Geometry: see drawing. Coordinates: mm, zero at the bounding-box minimum. A direction names the side the tool comes from. Give positions to 0.01 mm unless a question says otherwise; leave off trailing zeros. Loops run counter-clockwise (first coordinate to the right, second up) from the corner with the lowest first, then second, coordinate; pieces in that order, holes last. Notation, with made-up numbers: (38.5, 75) -> (78.5, 75) arc R17 cw to (78.5, 108) -> close; hole circle Ø9 at (46.25, 75.5). An arc over 180 degrees is marked (long way). Return JSON: item names as keys, results as strings. Group by question number.
(1) Cut plane C-C on z = 1.2. Return loops of the section in (x, y) (1 decimal), then the cut area to 3 significant figures.
(2) Cut plane D-D on x = 3.5. Return loops of the section in (y, z), then the cut area to 3 significant figures.
(3) Cut plane A-A on y = 21. Return loops of the section in (x, z) (1 decimal).
(4) Cut plane B-B on x = 24. Return loops of the section in (y, z) (1 decimal).
(5) Access query for the marked faces 1, 2, 3 and 4. Directions: +Z, -Z, +X, -X, +Y, -Y. A direction counts if a zero-diameter tool reaches every point of the face in a straight line with its end or side. Return the directions, or none.
(6) Draft query along X for the marked faces 5 and 6. Return one class per face: released by +X, released by -X, zero draft, split by the parting line, or undercut.
(7) Ray query, line 1 (Y direction, x = 9, z = 1); line 2 (X direction, y = 11.5, z = 1.8); line 3 (X direction, y = 7.5, z = 2.55) (1 decimal). Return the intervals inside material, ascending. Write a range as from..to.
(8) Pin query (flat end, axial travel): pin 1 (1.5 mm diameter, centred on x = 2, z = 2, fed in from +Y); pin 2 (1.5 mm diameter, centred on x = 9.5, z = 2, fed in from +Y); pin 3 (1.8 mm diameter, centred on x = 9.13, y = 6.13, fed in from -Z); pin 4 (1.5 mm diameter, centred on x = 2, z = 1, fed in from -Y). Return the tip coordinate at first contact, or that it passes through.
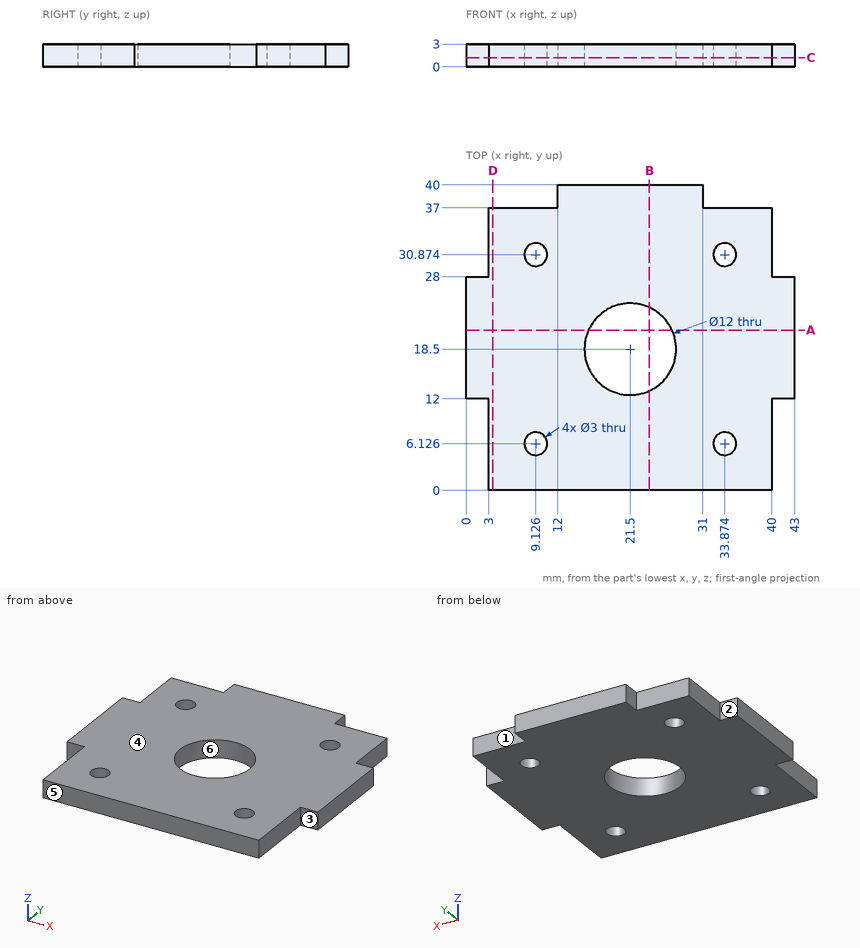
Answers:
{
 "1": {"outline": "(0, 12) -> (3, 12) -> (3, 0) -> (40, 0) -> (40, 12) -> (43, 12) -> (43, 28) -> (40, 28) -> (40, 37) -> (31, 37) -> (31, 40) -> (12, 40) -> (12, 37) -> (3, 37) -> (3, 28) -> (0, 28) -> close; hole circle Ø3 at (9.1, 6.1); hole circle Ø3 at (9.1, 30.9); hole circle Ø12 at (21.5, 18.5); hole circle Ø3 at (33.9, 6.1); hole circle Ø3 at (33.9, 30.9)", "area": "1,380 mm²"},
 "2": {"outline": "(0, 0) -> (37, 0) -> (37, 3) -> (0, 3) -> close", "area": "111 mm²"},
 "3": {"outline": "(0, 0) -> (16, 0) -> (16, 3) -> (0, 3) -> close; (27, 0) -> (43, 0) -> (43, 3) -> (27, 3) -> close"},
 "4": {"outline": "(0, 0) -> (13, 0) -> (13, 3) -> (0, 3) -> close; (24, 0) -> (40, 0) -> (40, 3) -> (24, 3) -> close"},
 "5": {"face 1": "+Z, -Z, +X, +Y", "face 2": "+Z, -Z, -X, +Y", "face 3": "+Z, -Z, +X, -Y", "face 4": "+Z, +X, -X, +Y, -Y"},
 "6": {"face 5": "zero draft", "face 6": "undercut"},
 "7": {"line 1": "0..4.63, 7.62..29.38, 32.37..37", "line 2": "3..40", "line 3": "3..8.5, 9.7..33.3, 34.5..40"},
 "8": {"pin 1": "y = 28", "pin 2": "y = 37", "pin 3": "through", "pin 4": "y = 12"}
}
